Geometry: final body of the model. Coordinates: model frame, mm. A direction names the side the tool comes from. Give positions to 0.01 mm unless a question says otherwise; leave off trailing zeros. Write each loop counter-clockwise with the first axis right and the second up, starting at its lowest first coordinate (ties: lowest second). Pieces come first, ordered by that corner, then holes. Notation, with made-up numbers: M 48.5,-31.75 L 68.5,-31.75 A23 ccw 68.5,-1.75 Z; hole C 55.5,-24 d5. An arc over 180 degrees is marked long. Use a Markdown table: item, result. Add a question column.
1) Pin query (flat end, axial travel): pin 1 (1 mm diameter, centred on x = -8.5, y = 21, fed in from -Z); pin 2 (10 mm diameter, centred on y = 48.5, z = -8, fed in from +X); pin 3 (4 mm diameter, centred on y = 50.5, z = -0.5, fed in from +X). Return the tip coordinate at first contact, or that it passes through.
2) Line query: line 1 (X direction, y = 1, z = -14); line 2 (Z direction, x = -20, y = 2.8); line 3 (X direction, y = 43.35, z = 0). Output: solid intervals per line, ascending.
3) Draft query along X for faces 6 (the flat face through (5.2, 2, 0)), 7 (the cylindrical face through (1.26, 49.42, -6.89)), 8 (the flat face through (3, 47, 8.7)). Return one class per face: +X half, -X half, draft (parallel to the pull), parting line (faces both ways), or undercut.
4) Section A-A on y = 19. Return the cut outline in (x, z).
5) Set-up query: faces 1 (the cylindrical face through (26.7, 2.38, 10.46)), 2 (the flat face through (4, 50, -6.7)), 3 (the conical face through (5.95, 0.58, -8.9)), 4 (the cylindrical face through (-16.736, 22.759, 10.324)), 5 (the cylindrical face through (-26.74, 2.42, 10.5)). Return all of +Z, -Z, +X, -X, +Y, -Y with unobstructed straight access to the full face (end or side cutting, diameter ignored); none if empty.
```python
from build123d import *

# Parameters (mm, degrees)
SKETCH5_R                = 13.8
BOSS_EXTRUDE10_DEPTH     = 55
BOSS_EXTRUDE13_DEPTH     = 13
SKETCH7_W                = 55.2
SKETCH7_H                = 37
BOSS_EXTRUDE11_DEPTH     = 4
SKETCH14_R               = 9.6
CUT_EXTRUDE9_DEPTH       = 53.773193953
FILLET1_R                = 1
FILLET3_R                = 3
CUT_EXTRUDE11_DEPTH      = 65.257373118
CUT_EXTRUDE11_DEPTH_BACK = 65.257373118
SKETCH2_R                = 2.25
CUT_EXTRUDE12_DEPTH      = 11
CHAMFER1_SIZE            = 0.8
FILLET7_R                = 1
SKETCH16_R               = 4.75
CUT_EXTRUDE13_DEPTH      = 56.136285693
SKETCH17_R               = 1.6
CUT_EXTRUDE14_DEPTH      = 3
FILLET8_R                = 2
DRAFT1_ANGLE             = 45


with BuildPart() as part:
    # Sketch5 → Boss-Extrude10 (new body)
    with BuildSketch(Plane(origin=(0, 55, 0), x_dir=(1, 0, 0), z_dir=(0, 1, 0))):
        with Locations((-8.6, 0)):
            Circle(SKETCH5_R)
    extrude(amount=-BOSS_EXTRUDE10_DEPTH)

    # Sketch5<9> → Boss-Extrude13 (add)
    with BuildSketch(Plane(origin=(0, 55, 0), x_dir=(1, 0, 0), z_dir=(0, 1, 0))):
        with BuildLine():
            Line((5.2, -8.7), (5.2, 8.4e-08))
            ThreePointArc((5.2, 8.4e-08), (4.405144544, -4.615865618), (2.112142643, -8.7))
            Line((2.112142643, -8.7), (5.2, -8.7))
        make_face()
        with BuildLine():
            Line((5.2, 8.4e-08), (5.2, 8.7))
            Line((5.2, 8.7), (2.112142643, 8.7))
            ThreePointArc((2.112142643, 8.7), (4.405144516, 4.615865697), (5.2, 8.4e-08))
        make_face()
    extrude(amount=-BOSS_EXTRUDE13_DEPTH)

    # Sketch7 → Boss-Extrude11 (add)
    with BuildSketch(Plane(origin=(0, 0, 0), x_dir=(1, 0, 0), z_dir=(0, 1, 0))):
        Rectangle(SKETCH7_W, SKETCH7_H)
    extrude(amount=BOSS_EXTRUDE11_DEPTH)

    # Sketch14 → Cut-Extrude9 (cut, through all)
    with BuildSketch(Plane(origin=(0, 41, 0), x_dir=(1, 0, 0), z_dir=(0, 1, 0))):
        with BuildLine():
            Line((-28.6, -9.6), (-8.6, -9.6))
            ThreePointArc((-8.6, -9.6), (-18.2, 0), (-8.6, 9.6))
            Line((-8.6, 9.6), (-28.6, 9.6))
            Line((-28.6, 9.6), (-28.6, -9.6))
        make_face()
        with Locations((-8.6, 0)):
            Circle(SKETCH14_R)
        Polygon((5.2, -9.6), (27.6, -9.6), (27.6, 9.6), (5.2, 9.6), (5.2, 0), align=None)
    extrude(amount=-CUT_EXTRUDE9_DEPTH, mode=Mode.SUBTRACT)

    # Fillet1
    fillet1_edges = [part.edges().sort_by_distance(p)[0] for p in [
        (-18.513626985, 22.5, -9.6),
        (-18.513626985, 22.5, 9.6),
    ]]
    fillet(fillet1_edges, radius=FILLET1_R)

    # Fillet3
    fillet3_edges = [part.edges().sort_by_distance(p)[0] for p in [
        (27.6, 2, -18.5),
        (-27.6, 2, -18.5),
        (-27.6, 2, 18.5),
        (27.6, 2, 18.5),
        (-27.6, 2, -9.6),
        (-27.6, 2, 9.6),
        (5.2, 2, 9.6),
        (5.2, 2, -9.6),
        (27.6, 2, -9.6),
        (27.6, 2, 9.6),
    ]]
    fillet(fillet3_edges, radius=FILLET3_R)

    # Sketch2 → Cut-Extrude11 (cut, two sides: drawn at the far end of the back side and taken through both)
    with BuildSketch(Plane(origin=(0, 0, 0), x_dir=(1, 0, 0), z_dir=(0, 1, 0)).offset(-CUT_EXTRUDE11_DEPTH_BACK)):
        with Locations(Location((-20, 14, 0), (0, 0, 270))):
            Circle(SKETCH2_R)
        with Locations(Location((20, 14, 0), (0, 0, 270))):
            Circle(SKETCH2_R)
        with Locations(Location((20, -14, 0), (0, 0, 270))):
            Circle(SKETCH2_R)
        with Locations(Location((-20, -14, 0), (0, 0, 270))):
            Circle(SKETCH2_R)
    extrude(amount=CUT_EXTRUDE11_DEPTH + CUT_EXTRUDE11_DEPTH_BACK, mode=Mode.SUBTRACT)

    # Sketch15 → Cut-Extrude12 (cut)
    with BuildSketch(Plane(origin=(0, 55, 0), x_dir=(1, 0, 0), z_dir=(0, 1, 0))):
        with BuildLine():
            Line((4.1, -6.7), (5.2, -6.7))
            Line((5.2, -6.7), (5.2, 6.7))
            Line((5.2, 6.7), (4.1, 6.7))
            Line((4.1, 6.7), (1.113392816, 6.7))
            ThreePointArc((1.113392816, 6.7), (-20.4, 0), (1.113392816, -6.7))
            Line((1.113392816, -6.7), (4.1, -6.7))
        make_face()
    extrude(amount=-CUT_EXTRUDE12_DEPTH, mode=Mode.SUBTRACT)

    # Chamfer1
    chamfer1_edges = [part.edges().sort_by_distance(p)[0] for p in [
        (16.4, 0, -9.6),
        (27.6, 0, -14.05),
        (-27.6, 0, -14.05),
        (0, 0, -18.5),
        (5.2, 0, 0),
        (16.4, 0, 9.6),
        (27.6, 0, 14.05),
        (0, 0, 18.5),
        (-27.6, 0, 14.05),
        (-26.721320344, 0, 17.621320344),
        (26.721320344, 0, 17.621320344),
        (26.721320344, 0, -17.621320344),
        (-26.721320344, 0, -17.621320344),
        (-26.721320344, 0, -10.478679656),
        (-26.721320344, 0, 10.478679656),
        (26.721320344, 0, 10.478679656),
        (26.721320344, 0, -10.478679656),
        (6.078679656, 0, -8.721320344),
        (6.078679656, 0, 8.721320344),
        (-16.6, 0, 9.6),
        (-16.6, 0, -9.6),
        (1, 0, 0),
    ]]
    chamfer(chamfer1_edges, length=CHAMFER1_SIZE)

    # Fillet7
    fillet7_edges = [part.edges().sort_by_distance(p)[0] for p in [
        (5.2, 48.5, 8.7),
        (2.112142643, 48.5, 8.7),
        (2.112142643, 48.5, -8.7),
        (5.2, 48.5, -8.7),
    ]]
    fillet(fillet7_edges, radius=FILLET7_R)

    # Sketch16 → Cut-Extrude13 (cut, through all)
    with BuildSketch(Plane(origin=(0, 44, 0), x_dir=(1, 0, 0), z_dir=(0, 1, 0))):
        with Locations(Location((-8.6, 0, 0), (0, 0, 270))):
            Circle(SKETCH16_R)
    extrude(amount=-CUT_EXTRUDE13_DEPTH, mode=Mode.SUBTRACT)

    # Sketch17 → Cut-Extrude14 (cut)
    with BuildSketch(Plane(origin=(0, 44, 0), x_dir=(1, 0, 0), z_dir=(0, 1, 0))):
        with Locations(Location((-8.6, 10, 0), (0, 0, 270))):
            Circle(SKETCH17_R)
    extrude(amount=-CUT_EXTRUDE14_DEPTH, mode=Mode.SUBTRACT)

    # Fillet8
    fillet8_edges = [part.edges().sort_by_distance(p)[0] for p in [
        (1.113392816, 49.5, -6.7),
        (1.113392816, 49.5, 6.7),
    ]]
    fillet(fillet8_edges, radius=FILLET8_R)

    # Draft1
    draft1_faces = [part.faces().sort_by_distance(p)[0] for p in [
        (4.269454108, 42, -6.535437948),
        (4.269454108, 42, 6.535437948),
    ]]
    draft(draft1_faces, Plane(origin=(5.2, 42, 0), x_dir=(0, 0, 1), z_dir=(1, 0, 0)), DRAFT1_ANGLE)


solid = part.part
```
Found:
| question | item | result |
|---|---|---|
| 1 | pin 1 | z = -13.8 |
| 1 | pin 2 | x = 5.2 |
| 1 | pin 3 | x = -20.13 |
| 2 | line 1 | -27.6 to -22.25, -17.75 to 17.75, 22.25 to 27.6 |
| 2 | line 2 | -18.5 to -16.25, -11.75 to -9.6, 9.6 to 11.75, 16.25 to 18.5 |
| 2 | line 3 | -22.4 to -13.35, -3.85 to 5.2 |
| 3 | face 6 | +X half |
| 3 | face 7 | undercut |
| 3 | face 8 | draft |
| 4 | outline | M -16.34,-11.43 A13.8 ccw long -16.34,11.43 A1 ccw -15.77,9.6 L -8.6,9.6 A9.6 cw -8.6,-9.6 L -15.77,-9.6 A1 ccw Z |
| 5 | face 1 | +X, +Y, -Y |
| 5 | face 2 | +X, +Y |
| 5 | face 3 | +X, -Y |
| 5 | face 4 | -X |
| 5 | face 5 | -X, +Y, -Y |
